CAD build for the part. Positions are in the model's coordinates, mm. A direction names the side the tool comes from. Give positions to 0.01 mm unless a question says otherwise; leave off trailing zeros. Order: outer loops, then holes, each group sorted by start corner. A loop starts at its lowest first (then second) coordinate and runs counter-clockwise, first axis right, second up. Notation, with made-up numbers: (-7, 59.5) -> (17, 59.5) arc R18 cw to (17, 66.5) -> close; hole circle Ø7 at (81.25, 67.5). An arc over 180 degrees is marked (long way). Use one line per item in the form item = value. Start each with the question number.
1) Cut at B-B, the plane y = 5. Give the cut face in (x, z).
2) Cut at A-A, the plane z = 13. Give the cut face in (x, y).
3) Mould opens along Y. For faces 6 (the face through (-34, 103.2, 28)), 7 (the face through (-62.834, 95.648, 52.697)), 8 (the face through (-68, 49, 28)) say: pulls with the +Y half, pulls with the -Y half, needs draft (parallel to the pull), parting line crosses it, or undercut.
4) Tool access for faces 1 (the face through (-56.092, 5.601, 14.097)), 2 (the face through (-44, -12, 1.66)), 3 (the face through (-34, 49, 0)), 4 (the face through (-62, 94, 30)), 5 (the face through (-56, 86, 17.4)): list every direction of +Z, -Z, +X, -X, +Y, -Y with a clear straight run to the whole face (end or side of a thin tool).
5) Cut at D-D, the plane x = -36. Give the cut face in (y, z).
6) Cut at C-C, the plane z = 35. Give the cut face in (x, y), and give its area (3 significant figures).
7) Drop flat-ended pins along their axis: P1, Ø8, axis at x = -1.5, z = 12.5, coming from the -Y side; P2, Ø8, axis at x = -57, y = 4.5, coming from the +Z side; P3, Ø2, axis at y = 67.5, z = 38, coming from the +X side. Give the stop position or say it passes through.
8) Probe line 1 (Y direction, x = -58, z = 12.5); line 2 (Y direction, x = -62.4, z = 52.75); line 3 (Z direction, x = 1.5, y = 76.5). List the from-to ranges inside material, lowest first.
from build123d import *

# Parameters (mm, degrees)
SKETCH_1_W      = 63
SKETCH_1_H      = 93
PAD_DEPTH       = 5
SKETCH_W        = 63
SKETCH_H        = 7.4
PAD001_DEPTH    = 5
PAD002_DEPTH    = 5
PAD003_DEPTH    = 51
SKETCH005_W     = 87.2
SKETCH005_H     = 1.4
PAD005_DEPTH    = 10
SKETCH006_R     = 3.6
PAD006_DEPTH    = 12.4
SKETCH007_R     = 2
POCKET001_DEPTH = 6.7
SKETCH008_W     = 44.6
SKETCH008_H     = 1.4
PAD007_DEPTH    = 10
PAD008_DEPTH    = 51
SKETCH010_W     = 7.2
SKETCH010_H     = 7.2
PAD009_DEPTH    = 51
SKETCH011_R     = 2
POCKET_DEPTH    = 6.7
FILLET_R        = 2


with BuildPart() as part:
    # Sketch_1 → Pad (new body)
    with BuildSketch(Plane.XY):
        with Locations((-31.5, 46.5)):
            Rectangle(SKETCH_1_W, SKETCH_1_H)
    extrude(amount=PAD_DEPTH)

    # Sketch → Pad001 (join)
    with BuildSketch(Plane.XY):
        with Locations((-31.5, -3.7)):
            Rectangle(SKETCH_W, SKETCH_H)
    extrude(amount=PAD001_DEPTH)

    # Sketch001 → Pad002 (join)
    with BuildSketch(Plane.XY):
        Polygon((-68, 103.2), (-68, -7.4), (-63, -7.4), (-63, 93), (0, 93), (0, 103.2), align=None)
    extrude(amount=PAD002_DEPTH)

    # Sketch002 (on Face13 of Pad002) → Pad003 (join)
    with BuildSketch(Plane.XY.offset(5)):
        Polygon((-68, 103.2), (-68, -7.4), (-66, -7.4), (-66, 101.2), (0, 101.2), (0, 103.2), align=None)
    extrude(amount=PAD003_DEPTH)

    # Sketch005 → Pad005 (join)
    with BuildSketch(Plane.YZ):
        with Locations((57.4, 2.36)):
            Rectangle(SKETCH005_W, SKETCH005_H)
    extrude(amount=PAD005_DEPTH)

    # Sketch006 (on Face11 of Pad005) → Pad006 (join)
    with BuildSketch(Plane.XY.offset(5)):
        with Locations((-58, 5)):
            Circle(SKETCH006_R)
        with Locations((-58, 88)):
            Circle(SKETCH006_R)
    extrude(amount=PAD006_DEPTH)

    # Sketch007 (on Face28 of Pad006) → Pocket001 (cut)
    with BuildSketch(Plane.XY.offset(17.4)):
        with Locations((-58, 5)):
            Circle(SKETCH007_R)
        with Locations((-58, 88)):
            Circle(SKETCH007_R)
    extrude(amount=-POCKET001_DEPTH, mode=Mode.SUBTRACT)

    # Sketch008 (on Face5 of Pocket001) → Pad007 (join)
    with BuildSketch(Plane.XZ.offset(7.4)):
        with Locations((-43.5, 2.36)):
            Rectangle(SKETCH008_W, SKETCH008_H)
    extrude(amount=PAD007_DEPTH)

    # Sketch009 (on Face21 of Pad007) → Pad008 (join)
    with BuildSketch(Plane.XY.offset(5)):
        Polygon((-65, -5.4), (-65, -8.9), (-66, -8.9), (-66, -5.4), (-66, -4.4), align=None)
    extrude(amount=PAD008_DEPTH)

    # Sketch010 (on Face22 of Pad008) → Pad009 (join)
    with BuildSketch(Plane.XY.offset(5)):
        with Locations((-62.4, 97.6)):
            Rectangle(SKETCH010_W, SKETCH010_H)
    extrude(amount=PAD009_DEPTH)

    # Sketch011 (on Face43 of Pad009) → Pocket (cut)
    with BuildSketch(Plane.XY.offset(56)):
        with Locations((-62.4, 97.6)):
            Circle(SKETCH011_R)
    extrude(amount=-POCKET_DEPTH, mode=Mode.SUBTRACT)

    # Fillet
    fillet_edges = [part.edges().sort_by_distance(p)[0] for p in [
        (-61.6, 5, 5),
        (-61.6, 88, 5),
    ]]
    fillet(fillet_edges, radius=FILLET_R)


solid = part.part
Result:
q1.outline = (-68, 0) -> (0, 0) -> (0, 5) -> (-52.4, 5) arc R2 cw to (-54.4, 7) -> (-54.4, 17.4) -> (-56, 17.4) -> (-56, 10.7) -> (-60, 10.7) -> (-60, 17.4) -> (-61.6, 17.4) -> (-61.6, 7) arc R2 cw to (-63.6, 5) -> (-66, 5) -> (-66, 56) -> (-68, 56) -> close
q2.outline = (-68, -7.4) -> (-66, -7.4) -> (-66, -8.9) -> (-65, -8.9) -> (-65, -5.4) -> (-66, -4.4) -> (-66, 94) -> (-58.8, 94) -> (-58.8, 101.2) -> (0, 101.2) -> (0, 103.2) -> (-68, 103.2) -> close; circle Ø7.2 at (-58, 5); circle Ø7.2 at (-58, 88); hole circle Ø4 at (-58, 5); hole circle Ø4 at (-58, 88)
q3.face_6 = pulls with the +Y half
q3.face_7 = undercut
q3.face_8 = needs draft
q4.face_1 = +Z
q4.face_2 = -Z, +X, -X, -Y
q4.face_3 = -Z, +X, -X, +Y, -Y
q4.face_4 = +Z, +X
q4.face_5 = +Z, +X, -Y
q5.outline = (-17.4, 1.66) -> (-7.4, 1.66) -> (-7.4, 0) -> (103.2, 0) -> (103.2, 56) -> (101.2, 56) -> (101.2, 5) -> (-7.4, 5) -> (-7.4, 3.06) -> (-17.4, 3.06) -> close
q6.outline = (-68, -7.4) -> (-66, -7.4) -> (-66, -8.9) -> (-65, -8.9) -> (-65, -5.4) -> (-66, -4.4) -> (-66, 94) -> (-58.8, 94) -> (-58.8, 101.2) -> (0, 101.2) -> (0, 103.2) -> (-68, 103.2) -> close
q6.area = 409 mm²
q7.P1 = 101.2
q7.P2 = 17.4
q7.P3 = -66
q8.line_1 = 1.4 to 3, 7 to 8.6, 84.4 to 86, 90 to 91.6, 101.2 to 103.2
q8.line_2 = 94 to 95.6, 99.6 to 103.2
q8.line_3 = 1.66 to 3.06
